Verification items for the finished model (mm, model axes). A direction names the side the tool comes from. Coordinates: 2 decimals unless noted, no trailing zeros. Order: outer loops, then holes, each group sorted by start corner. A loop starts at its lowest first (then second) coordinate and runs counter-clockwise, first axis right, second up.
Q1. Depth check by flat-ended pin: P1, Ø0.5, axis at y = -2, z = 0.5, coming from the -X side. Enter the tip coordinate at first touch or a pass-through.
Q2. Cross-section at B-B, the plane x = -13.5. Record the boundary of the cut face in (y, z), and give its area (3 significant figures).
Q3. Draft check along Y on faces 4 (the cylindrical face through (-5.05, 4.23, 0.78)), 5 (the flat face through (-23.95, 13, 1)), 6 (the cylindrical face through (23.05, 24.14, 0.8)). Enter one of: pulls with the +Y half, pulls with the -Y half, needs draft (parallel to the pull), parting line crosses it, or undercut.
Q4. Cross-section at C-C, the plane z = 1.3. Count the separate pieces of the cut face and the enclosed holes in it, and give its area (3 significant figures).
Q5. Thickness scan on line 1 (Y direction, x = 2.5, z = 0.65); line 2 (Y direction, x = -13.5, z = 1.15); line 3 (X direction, y = 13, z = 0.1). Record the ranges inside material, lowest first.
Q6. Cross-section at D-D, the plane x = 18.5. Record the boundary of the cut face in (y, z), and give its area (3 significant figures).
Q7. Cross-section at A-A, the plane y = 13.25. Record the boundary of the cut face in (x, z), and give its area (3 significant figures).
Q8. Set-up check for faces 1 (the cylindrical face through (4.7, 7.3, 0.8)), 2 (the flat face through (4.95, -3, 1)), 3 (the flat face through (0, 25, 1)): record each of +Z, -Z, +X, -X, +Y, -Y from which the full face is reachable in a straight line by a thin tool's end or side.
from build123d import *

# Parameters (mm, degrees)
F2_R     = 8.25
F2_W     = 9.9
F2_H     = 6.6
F3_DEPTH = 1.5875
F4_W     = 11
F4_H     = 4.4
F4_W_2   = 10.5
F4_H_2   = 2
F5_DEPTH = 1.5885
F6_R     = 3
F7_R     = 2.19999


# Not quite as in the source:
# - a fillet or chamfer is up to 0.001 mm smaller than in the source, because OpenCascade refuses the exact size


with BuildPart() as f3:
    # F2 (on Top) → F3 (new body)
    with BuildSketch(Plane.XY):
        Polygon((-23.95, 25), (-23.95, 0), (-4.95, 0), (4.95, 0), (23.95, 0), (23.95, 25), align=None)
        with Locations((-13.5, 13.25)):
            Circle(F2_R, mode=Mode.SUBTRACT)
        with Locations((12.4, 13.25)):
            Circle(F2_R, mode=Mode.SUBTRACT)
        with Locations((0, -3.3)):
            Rectangle(F2_W, F2_H)
    extrude(amount=F3_DEPTH)

    # F4 (on face) → F5 (cut, through all)
    with BuildSketch(Plane.XY.offset(1.5875)):
        with Locations((-0.2067205198, 5.8)):
            Rectangle(F4_W, F4_H)
        with Locations((-0.3, 21.9)):
            Rectangle(F4_W_2, F4_H_2)
    extrude(amount=-F5_DEPTH, mode=Mode.SUBTRACT)

    # F6
    f6_edges = [f3.edges().sort_by_distance(p)[0] for p in [
        (-23.95, 0, 0.79375),
        (-23.95, 25, 0.79375),
        (23.95, 25, 0.79375),
        (23.95, 0, 0.79375),
    ]]
    fillet(f6_edges, radius=F6_R)

    # F7 (radius 2.2 in the source; OpenCascade refuses exactly that, so slightly less here)
    f7_edges = [f3.edges().sort_by_distance(p)[0] for p in [
        (-5.706721, 3.6, 0.79375),
        (-5.706721, 8, 0.79375),
        (5.293279, 3.6, 0.79375),
        (5.293279, 8, 0.79375),
    ]]
    fillet(f7_edges, radius=F7_R)


solid = f3.part
Check values:
1. P1: stops at x = -4.95
2. outline: (0, 0) - (5, 0) - (5, 1.59) - (0, 1.59) - close; (21.5, 0) - (25, 0) - (25, 1.59) - (21.5, 1.59) - close
2. area: 13.5 mm2
3. face 4: undercut
3. face 5: needs draft
3. face 6: pulls with the +Y half
4. separate pieces: 1
4. enclosed holes: 4
4. area: 762 mm2
5. line 1: y = -6.6 to 3.6, 8 to 20.9, 22.9 to 25
5. line 2: y = 0 to 5, 21.5 to 25
5. line 3: x = -23.95 to -21.75, -5.25 to 4.15, 20.65 to 23.95
6. outline: (0, 0) - (7.7, 0) - (7.7, 1.59) - (0, 1.59) - close; (18.8, 0) - (25, 0) - (25, 1.59) - (18.8, 1.59) - close
6. area: 22.1 mm2
7. outline: (-23.95, 0) - (-21.75, 0) - (-21.75, 1.59) - (-23.95, 1.59) - close; (-5.25, 0) - (4.15, 0) - (4.15, 1.59) - (-5.25, 1.59) - close; (20.65, 0) - (23.95, 0) - (23.95, 1.59) - (20.65, 1.59) - close
7. area: 23.7 mm2
8. face 1: +Z, -Z
8. face 2: +Z, -Z, +X, -Y
8. face 3: +Z, -Z, +X, -X, +Y
